Design review of the part built by this model. Coordinates are the model's own, in mm. A direction names the side the tool comes from. Round coordinates to 2 decimals unless told otherwise and drop trailing zeros. Loops run counter-clockwise (first coordinate to the right, second up) from the corner with the lowest first, then second, coordinate; pieces in that order, holes last. Notation, with made-up numbers: M 40.5,34 L 93.5,34 A23 ccw 93.5,51 Z; hole C 36,62.25 d11. An arc over 180 degrees is marked long. Use a Markdown table: item, result.
from build123d import *

# Parameters (mm, degrees)
SKETCH1_R           = 0.5
BOSS_EXTRUDE2_DEPTH = 30
SKETCH9_R           = 0.5
BOSS_EXTRUDE3_DEPTH = 5


with BuildPart() as part:
    # Sketch1 → Boss-Extrude2 (new body)
    with BuildSketch(Plane(origin=(0, 0, 0), x_dir=(1, 0, 0), z_dir=(0, 1, 0))):
        with Locations(Location((0, 0, 0), (0, 0, 270))):
            Circle(SKETCH1_R)
    extrude(amount=BOSS_EXTRUDE2_DEPTH)

    # Sketch9 → Boss-Extrude3 (add)
    with BuildSketch(Plane(origin=(0, 0, 0), x_dir=(0, 0, -1), z_dir=(1, 0, 0))):
        Circle(SKETCH9_R)
        with Locations((0, 30)):
            Circle(SKETCH9_R)
    extrude(amount=BOSS_EXTRUDE3_DEPTH)


solid = part.part
1. Machinability: for faces 3 (the face through (2.5, 30.4, -0.3)), 4 (the face through (-0.488, 14.79, -0.108)), 5 (the face through (5, 0, 0)), which of the approach directions +Z, -Z, +X, -X, +Y, -Y give a long, thin tool a straight path to every point of the face, cutting with its end or side? Answer none if there is none.
Check values:
| item | result |
|---|---|
| face 3 | +X |
| face 4 | none |
| face 5 | +Z, -Z, +X, +Y, -Y |
2. Take a section at C-C on y = 15.5. Give the boundary of the cut face in (x, z), and give its area (3 significant figures).
Check values:
| item | result |
|---|---|
| outline | C 0,0 d1 |
| area | 0.785 mm² |
3. Take a section at B-B on x = 1.45. Give the boundary of the cut face in (y, z), and give its area (3 significant figures).
Check values:
| item | result |
|---|---|
| outline | C 0,0 d1; C 30,0 d1 |
| area | 1.57 mm² |
4. Take a section at A-A on z = 0.3. Give the boundary of the cut face in (x, y), and give its area (3 significant figures).
Check values:
| item | result |
|---|---|
| outline | M -0.4,0 L 0,0 L 0,-0.4 L 5,-0.4 L 5,0.4 L 0.4,0.4 L 0.4,29.6 L 5,29.6 L 5,30.4 L 0,30.4 L 0,30 L -0.4,30 Z |
| area | 31.7 mm² |
5. Wall thickness on line 1 along Y through (x, z) = (3.3, 0.05); line 2 along X through (y, z) = (24, 0.05); line 3 along Y through (x, z) = (2.3, -0.3): over which ranges is each line inside the solid? List them lowest first. Write a range as from..to.
Check values:
| item | result |
|---|---|
| line 1 | y = -0.5..0.5, 29.5..30.5 |
| line 2 | x = -0.5..0.5 |
| line 3 | y = -0.4..0.4, 29.6..30.4 |
6. The part is to be moulded in two halves that separate along Y. For faces 1 (the face through (5, 30, 0)), 2 (the face through (2.465, -0.444, -0.231)), say which applies: pulls with the +Y half, pulls with the -Y half, needs draft (parallel to the pull), parting line crosses it, or undercut.
Check values:
| item | result |
|---|---|
| face 1 | needs draft |
| face 2 | undercut |
